```python
from build123d import *

# Parameters (mm, degrees)
SKETCH_1_W      = 12
SKETCH_1_H      = 12
SKETCH_1_W_2    = 7
SKETCH_1_H_2    = 3
SKETCH_1_R      = 1
EXTRUDE_1_DEPTH = 0.4
EXTRUDE_START   = 0.4
SKETCH_1_5_R    = 2.5
EXTRUDE_2_DEPTH = 1.6
SKETCH_1_6_R    = 5
EXTRUDE_3_DEPTH = 0.01
FILLET_1_R      = 1.5


with BuildPart() as part:
    # 草图1 → 凸台-拉伸1 (new body)
    # profile 1 of 2: a face of its own
    with BuildSketch(Plane(origin=(0, 0, 0), x_dir=(1, 0, 0), z_dir=(0, 1, 0))):
        Rectangle(SKETCH_1_W, SKETCH_1_H)
    # profile 2 of 2: a face of its own
    with BuildSketch(Plane(origin=(0, 0, 0), x_dir=(1, 0, 0), z_dir=(0, 1, 0))):
        with Locations((-9.5, 0)):
            Rectangle(SKETCH_1_W_2, SKETCH_1_H_2)
        with Locations(Location((-11.5, 0, 0), (0, 0, 270))):
            Circle(SKETCH_1_R, mode=Mode.SUBTRACT)
    extrude(amount=EXTRUDE_1_DEPTH)

    # 草图1<5> → 凸台-拉伸2 (add)
    with BuildSketch(Plane(origin=(0, 0, 0), x_dir=(1, 0, 0), z_dir=(0, 1, 0)).offset(EXTRUDE_START)):
        with Locations(Location((0, 0, 0), (0, 0, 90))):
            Circle(SKETCH_1_5_R)
    extrude(amount=EXTRUDE_2_DEPTH)

    # 草图1<6> → 凸台-拉伸3 (add)
    with BuildSketch(Plane(origin=(0, 0, 0), x_dir=(1, 0, 0), z_dir=(0, 1, 0)).offset(EXTRUDE_START)):
        with Locations(Location((0, 0, 0), (0, 0, 90))):
            Circle(SKETCH_1_6_R)
    extrude(amount=EXTRUDE_3_DEPTH)

    # loft up to a face of the part (loft_1)
    loft([Face(Wire([part.edges().sort_by_distance((-1.822421569, 2, 1.711367765))[0]])), Face(Wire([part.edges().sort_by_distance((-3.644843137, 0.4, 3.42273553))[0]]))])

    # 圆角1
    fillet_1_edges = [part.edges().sort_by_distance(p)[0] for p in [
        (-13, 0.2, 1.5),
        (-13, 0.2, -1.5),
    ]]
    fillet(fillet_1_edges, radius=FILLET_1_R - 0.0001)  # a hair under: the kernel refuses the full size


solid = part.part
```
CAD build for the part. Positions are in the model's coordinates, mm. A direction names the side the tool comes from. Round coordinates to 2 decimals unless told otherwise and drop trailing zeros. Write each loop counter-clockwise with the first axis right and the second up, starting at its lowest first coordinate (ties: lowest second). Pieces come first, ordered by that corner, then holes. Notation, with made-up numbers: (-2, 27.5) - (22, 27.5) arc R11 cw to (22, 40.5) - close; hole circle Ø10 at (39.5, 51). An arc over 180 degrees is marked (long way). Write item = value, one per line. Start each with the question number.
Q1. Which spindle directions (+Z, -Z, +X, -X, +Y, -Y) get a long thin tool onto all of the face, cutting with end or side? Do faces 4 (the flat face through (0, 2, 0)), 5 (the flat face through (-6, 0.4, 0)). Say none if no direction does.
Q2. Band-saw the part on C-C (y = 0.75). Give the cut face in (x, z), then the cut area to 3 significant figures.
Q3. Band-saw the part on B-B (y = 1.8). Give the cut face in (x, z) (1 decimal), then the cut area to 3 significant figures.
Q4. Drop flat-ended pins along their axis: pin 1 (1.5 mm diameter, centred on x = 3.5, z = -4.5, fed in from +Y); pin 2 (1.5 mm diameter, centred on x = -9.5, z = 3.5, fed in from +Y). Give the stop position or say it passes through.
Q5. Mould opens along X. For faces 1 (the flat face through (-2, 0, 0)), 2 (the cylindrical face through (-12.55, 0.2, 1.07)), 3 (the cylindrical face through (-10.51, 0.2, -0.13)) say: pulls with the +X half, pulls with the -X half, needs draft (parallel to the pull), parting line crosses it, or undercut.
Q6. Band-saw the part on A-A (x = -6.5). Give the cut face in (y, z).
Q7. Probe L1, parallel to X at y = 0.2, z = 0; L2, parallel to Y at x = -4.75, z = -3; L3, parallel to X at y = 1.45, z = 1.75. List the from-to ranges inside material, lowest first. Write a range as from..to.
Answers below:
q1.face_4 = +Z, -Z, +X, -X, +Y
q1.face_5 = +Y
q2.outline = circle Ø8.91 at (0, 0)
q2.area = 62.3 mm2
q3.outline = circle Ø5.6 at (0, 0)
q3.area = 24.9 mm2
q4.pin_1 = 0.43
q4.pin_2 = through
q5.face_1 = needs draft
q5.face_2 = pulls with the -X half
q5.face_3 = undercut
q6.outline = (0, -1.5) - (0.4, -1.5) - (0.4, 1.5) - (0, 1.5) - close
q7.L1 = -13..-12.5, -10.5..6
q7.L2 = 0..0.4
q7.L3 = -2.87..2.87
